The listing builds one solid part. Answer for the finished solid, in the listing's coordinates (mm). A direction names the side the tool comes from. Coordinates: 2 decimals unless noted, no trailing zeros. Use one line per item in the form item = value. Start each with the question number.
Item 1: The mould has two halves that part along Z. Classify faces 1 (the cylindrical face through (30.623, 0.743, 59.587)), 2 (the flat face through (55, -7, 55.562)), 3 (the flat face through (47, 0, 63.5)): released by +Z, released by -Z, zero draft, split by the parting line, or undercut.
Item 2: A tool of negligible diameter and unlimited length cuts with its end or side. For faces 4 (the cylindrical face through (95.072, 1.256, 28.547)), 5 (the flat face through (19, 0, -46.99)), 6 (the cylindrical face through (3.447, -6.469, -43.077)), 7 (the flat face through (82.55, -17, -15)), 8 (the flat face through (138.176, 0, 0)), from which of +Z, -Z, +X, -X, +Y, -Y can it reach the whole face along a straight path? Write none if from no direction.
Item 3: Each of these flat-tipped pins is pushed along its axis until it touches: pin 1 Ø6 at (x, z) = (59, 11.5) entering from +Y; pin 2 Ø17 at (x, y) = (54.5, -3) entering from -Z (3 decimals); pin 3 Ø1.5 at (y, z) = (-12.5, 22.5) entering from +X. Where does it stop, or does it pass through?
Item 4: Consider line 1 along Z through (x, y) = (85.5, 1); line 2 along Z through (x, y) = (10, 8.5); line 3 along Z through (x, y) = (38, 2). Determine where each line is inside the solid, lowest interval first. Write a range as [from, to].
Item 5: Section D-D, the plane y = -15 is taken. Count the separate pieces of the cut face and the enclosed holes in it, and give its area (3 significant figures).
from build123d import *

# Parameters (mm, degrees)
SKETCH1_R      = 22.225
EXTRUDE1_DEPTH = 82.55
SKETCH2_R      = 9.525
EXTRUDE2_DEPTH = 63.5
SKETCH3_R      = 9.525
EXTRUDE3_DEPTH = 46.99
SKETCH4_R      = 16.891
EXTRUDE4_DEPTH = 7.9375
SKETCH5_R      = 16.891
EXTRUDE5_DEPTH = 7.9375
SKETCH6_R      = 28.575
EXTRUDE6_DEPTH = 25.4
SKETCH7_R      = 6.35
EXTRUDE7_DEPTH = 30.226
FILLET1_R      = 4.7625


with BuildPart() as part:
    # Sketch1 → Extrude1 (new body)
    with BuildSketch(Plane(origin=(0, 0, 0), x_dir=(0, 0, -1), z_dir=(1, 0, 0))):
        Circle(SKETCH1_R)
    extrude(amount=EXTRUDE1_DEPTH)

    # Sketch2 → Extrude2 (add)
    with BuildSketch(Plane.XY):
        with Locations((47.498, 0)):
            Circle(SKETCH2_R)
    extrude(amount=EXTRUDE2_DEPTH)

    # Sketch3 → Extrude3 (add)
    with BuildSketch(Plane.XY):
        with Locations((19.05, 0)):
            Circle(SKETCH3_R)
    extrude(amount=-EXTRUDE3_DEPTH)

    # Sketch4 → Extrude4 (add)
    with BuildSketch(Plane(origin=(0, 0, -46.99), x_dir=(-1, 0, 0), z_dir=(0, 0, -1))):
        with Locations((-19.05, 0)):
            Circle(SKETCH4_R)
    extrude(amount=-EXTRUDE4_DEPTH)

    # Sketch5 → Extrude5 (add)
    with BuildSketch(Plane.XY.offset(63.5)):
        with Locations((47.498, 0)):
            Circle(SKETCH5_R)
    extrude(amount=-EXTRUDE5_DEPTH)

    # Sketch6 → Extrude6 (add)
    with BuildSketch(Plane(origin=(82.55, 0, 0), x_dir=(0, 0, -1), z_dir=(1, 0, 0))):
        Circle(SKETCH6_R)
    extrude(amount=EXTRUDE6_DEPTH)

    # Sketch7 → Extrude7 (add)
    with BuildSketch(Plane(origin=(107.95, 0, 0), x_dir=(0, 0, -1), z_dir=(1, 0, 0))):
        Circle(SKETCH7_R)
    extrude(amount=EXTRUDE7_DEPTH)

    # Fillet1
    fillet1_edges = [part.edges().sort_by_distance(p)[0] for p in [
        (0, 0, 22.225),
    ]]
    fillet(fillet1_edges, radius=FILLET1_R)


solid = part.part
Response:
q1.face_1 = zero draft
q1.face_2 = undercut
q1.face_3 = released by +Z
q2.face_4 = +X
q2.face_5 = -Z, +X, -X, +Y, -Y
q2.face_6 = -Z
q2.face_7 = none
q2.face_8 = +Z, -Z, +X, +Y, -Y
q3.pin_1 = 20.54
q3.pin_2 = -22.225
q3.pin_3 = 107.95
q4.line_1 = [-28.56, 28.56]
q4.line_2 = [-46.99, -39.05], [-20.54, 20.54]
q4.line_3 = [-22.13, 22.13], [55.56, 63.5]
q5.separate_pieces = 3
q5.enclosed_holes = 0
q5.area = 4,180 mm2
